Geometry check sheet. Reference: drawing and pictorial views, mm from the part's lowest x, y, z. Give positions to 0.01 mm unless a question says otherwise; leave off trailing zeros. Order: outer loops, then holes, each group sorted by start corner. A loop starts at its lowest first (then second) coordinate and runs counter-clockwise, first axis right, second up. Notation, with made-up numbers: (-9.5, -15) - (8.5, -15) arc R28 ccw to (8.5, 7) - close; hole circle Ø4 at (56.5, 57). An arc over 180 degrees is marked (long way). Answer as a JSON object with one key per item and string values.
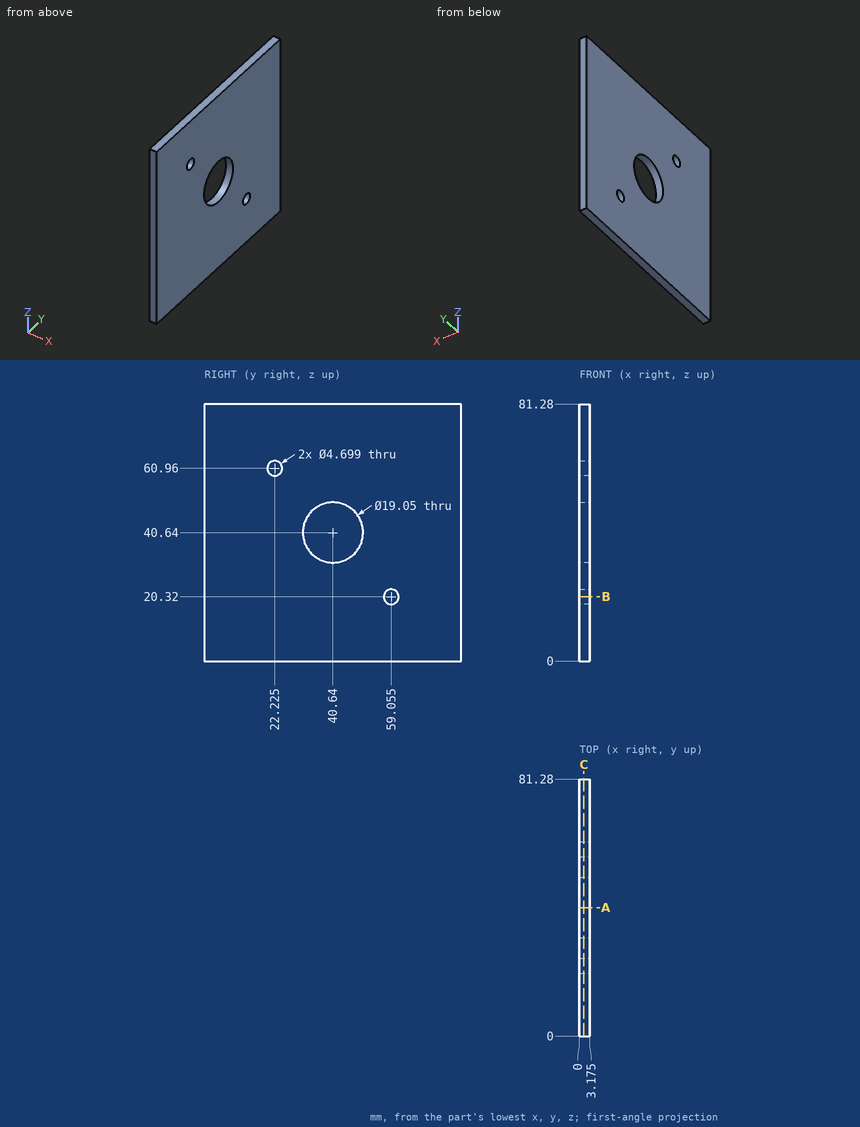
(1) Section check B-B (z = 20.32). Record the cut outline in (x, y) (1 decimal), then the cut area to 3 significant figures.
Computed values:
{"outline": "(0, 0) - (3.2, 0) - (3.2, 56.7) - (0, 56.7) - close; (0, 61.4) - (3.2, 61.4) - (3.2, 81.3) - (0, 81.3) - close", "area": "243 mm²"}
(2) Section check A-A (y = 40.64). Record the cut outline in (x, z) (3 decimals).
Computed values:
{"outline": "(0, 0) - (3.175, 0) - (3.175, 31.115) - (0, 31.115) - close; (0, 50.165) - (3.175, 50.165) - (3.175, 81.28) - (0, 81.28) - close"}
(3) Section check C-C (x = 1.4). Count the separate pieces of the cut face and the enclosed holes in it, then the cut area to 3 significant figures.
Computed values:
{"separate pieces": "1", "enclosed holes": "3", "area": "6,290 mm²"}
(4) Material ranges on line 1 along Y through (x, z) = (0.6, 60.96); line 2 along Y through (x, z) = (1.9, 20.32); line 3 along Z through (x, y) = (0.7, 49), recorded low to high. Write a range as [from, to].
Computed values:
{"line 1": "y = [0, 19.88], [24.57, 81.28]", "line 2": "y = [0, 56.71], [61.4, 81.28]", "line 3": "z = [0, 36.08], [45.2, 81.28]"}
